from build123d import *

# Parameters (mm, degrees)
SKETCH_W             = 95
SKETCH_H             = 48
PAD_DEPTH            = 2
SKETCH001_W          = 95
SKETCH001_H          = 48
SKETCH001_W_2        = 91
SKETCH001_H_2        = 44
PAD001_DEPTH         = 18.5
SKETCH002_W          = 43.5
SKETCH002_H          = 20.5
POCKET_DEPTH         = 5
SKETCH003_W          = 5
SKETCH003_H          = 20.5
PAD002_DEPTH         = 2
SKETCH004_R          = 0.7
POCKET001_DEPTH      = 3
SKETCH005_W          = 4.5
SKETCH005_H          = 2.7
SKETCH005_W_2        = 5.5
SKETCH005_W_3        = 20
SKETCH005_H_2        = 2
SKETCH005_W_4        = 12
SKETCH005_H_3        = 1
SKETCH005_W_5        = 2
PAD003_DEPTH         = 2.5
PAD004_DEPTH         = 17
SKETCH007_W          = 1
SKETCH007_H          = 2.7
POCKET002_DEPTH      = 14
SKETCH008_W          = 3.5
SKETCH008_H          = 9.5
POCKET003_DEPTH      = 2
SKETCH009_R          = 1
POCKET004_DEPTH      = 2
PAD005_DEPTH         = 4
SKETCH011_W          = 70
SKETCH011_H          = 3
SKETCH011_W_2        = 2
SKETCH011_H_2        = 3.5
SKETCH011_W_3        = 3
PAD006_DEPTH         = 15
SKETCH012_W          = 15
SKETCH012_H          = 12.85
PAD007_DEPTH         = 7.3
SKETCH013_W          = 12
SKETCH013_H          = 10.8
POCKET005_DEPTH      = 4
SKETCH014_W          = 5
SKETCH014_H          = 5
POCKET006_DEPTH      = 6
SKETCH015_R          = 3.2
POCKET007_DEPTH      = 5
POCKET007_DEPTH_BACK = 100
SKETCH017_R          = 1
POCKET008_DEPTH      = 10
SKETCH018_R          = 1.6
POCKET009_DEPTH      = 5
SKETCH019_R          = 1.6
POCKET010_DEPTH      = 5
SKETCH026_R          = 2.1
SKETCH026_R_2        = 2.5
POCKET014_DEPTH      = 5
FILLET003_R          = 2
FILLET004_R          = 1.95
CHAMFER001_SIZE      = 2
FILLET005_R          = 1
CHAMFER003_SIZE      = 1.2
CHAMFER004_SIZE      = 1.2
FILLET013_R          = 1
FILLET014_R          = 0.9
SKETCH049_W          = 3
SKETCH049_H          = 1
POCKET020_DEPTH      = 2.5
SKETCH050_W          = 5
SKETCH050_H          = 7
POCKET021_DEPTH      = 5


with BuildPart() as part:
    # Sketch → Pad (new body)
    with BuildSketch(Plane.XY):
        with Locations((47.5, 24)):
            Rectangle(SKETCH_W, SKETCH_H)
    extrude(amount=PAD_DEPTH)

    # Sketch001 (on Face6 of Pad) → Pad001 (join)
    with BuildSketch(Plane.XY.offset(2)):
        with Locations((47.5, 24)):
            Rectangle(SKETCH001_W, SKETCH001_H)
        with Locations((47.5, 24)):
            Rectangle(SKETCH001_W_2, SKETCH001_H_2, mode=Mode.SUBTRACT)
    extrude(amount=PAD001_DEPTH)

    # Sketch002 (on Face15 of Pad001) → Pocket (cut)
    with BuildSketch(Plane.XY.offset(2)):
        with Locations((66.25, 35.75)):
            Rectangle(SKETCH002_W, SKETCH002_H)
    extrude(amount=-POCKET_DEPTH, mode=Mode.SUBTRACT)

    # Sketch003 (on Face15 of Pocket) → Pad002 (join)
    with BuildSketch(Plane.XY.offset(2)):
        with Locations((42, 35.75)):
            Rectangle(SKETCH003_W, SKETCH003_H)
        with Locations((90.5, 35.75)):
            Rectangle(SKETCH003_W, SKETCH003_H)
    extrude(amount=PAD002_DEPTH)

    # Sketch004 (on Face26 of Pad002) → Pocket001 (cut)
    with BuildSketch(Plane.XY.offset(4)):
        with Locations((90.2, 43.6)):
            Circle(SKETCH004_R)
        with Locations((90.2, 28.6)):
            Circle(SKETCH004_R)
        with Locations((42, 43.6)):
            Circle(SKETCH004_R)
        with Locations((42, 28.6)):
            Circle(SKETCH004_R)
    extrude(amount=-POCKET001_DEPTH, mode=Mode.SUBTRACT)

    # Sketch005 (on Face16 of Pocket001) → Pad003 (join)
    with BuildSketch(Plane.XY.offset(2)):
        with Locations((4.25, 44.65)):
            Rectangle(SKETCH005_W, SKETCH005_H)
        with Locations((19.25, 44.65)):
            Rectangle(SKETCH005_W_2, SKETCH005_H)
        with Locations((12, 40.6)):
            Rectangle(SKETCH005_W_3, SKETCH005_H_2)
        with Locations((8, 37.35)):
            Rectangle(SKETCH005_W_4, SKETCH005_H_3)
        with Locations((21, 37.35)):
            Rectangle(SKETCH005_W_5, SKETCH005_H_3)
    extrude(amount=PAD003_DEPTH)

    # Sketch006 (on Face16 of Pad003) → Pad004 (join)
    with BuildSketch(Plane.XY.offset(2)):
        Polygon((30, 46), (33, 46), (33, 36.85), (27.6, 36.85), (27.6, 40.6), (30, 40.6), align=None)
    extrude(amount=PAD004_DEPTH)

    # Sketch007 (on Face13 of Pad004) → Pocket002 (cut)
    with BuildSketch(Plane.XY.offset(20.5)):
        with Locations((1.5, 44.65)):
            Rectangle(SKETCH007_W, SKETCH007_H)
    extrude(amount=-POCKET002_DEPTH, mode=Mode.SUBTRACT)

    # Sketch008 (on Face7 of Pocket002) → Pocket003 (cut)
    with BuildSketch(Plane(origin=(0, 0, 0), x_dir=(0, -1, 0), z_dir=(-1, 0, 0))):
        with Locations((-44.25, 10.25)):
            Rectangle(SKETCH008_W, SKETCH008_H)
    extrude(amount=-POCKET003_DEPTH, mode=Mode.SUBTRACT)

    # Sketch009 (on Face14 of Pocket003) → Pocket004 (cut)
    with BuildSketch(Plane(origin=(0, 48, 0), x_dir=(-1, 0, 0), z_dir=(0, 1, 0))):
        with Locations((-9.2, 3)):
            Circle(SKETCH009_R)
        with Locations((-13.7, 3)):
            Circle(SKETCH009_R)
    extrude(amount=-POCKET004_DEPTH, mode=Mode.SUBTRACT)

    # Sketch010 (on Face20 of Pocket004) → Pad005 (join)
    with BuildSketch(Plane.XY.offset(2)):
        Polygon((2, 35.5), (20.5, 35.5), (20.5, 2), (22.5, 2), (22.5, 36.85), (20, 36.85), (20, 35.85), (14, 35.85), (14, 36.85), (2, 36.85), align=None)
    extrude(amount=PAD005_DEPTH)

    # Sketch011 (on Face20 of Pad005) → Pad006 (join)
    with BuildSketch(Plane.XY.offset(2)):
        with Locations((58, 22.5)):
            Rectangle(SKETCH011_W, SKETCH011_H)
        with Locations((92, 3.75)):
            Rectangle(SKETCH011_W_2, SKETCH011_H_2)
        with Locations((92, 19.25)):
            Rectangle(SKETCH011_W_2, SKETCH011_H_2)
        with Locations((24.5, 19.25)):
            Rectangle(SKETCH011_W_3, SKETCH011_H_2)
        with Locations((24.5, 3.75)):
            Rectangle(SKETCH011_W_3, SKETCH011_H_2)
    extrude(amount=PAD006_DEPTH)

    # Sketch012 (on Face20 of Pad006) → Pad007 (join)
    with BuildSketch(Plane.XY.offset(2)):
        with Locations((30, 30.425)):
            Rectangle(SKETCH012_W, SKETCH012_H)
    extrude(amount=PAD007_DEPTH)

    # Sketch013 (on Face73 of Pad007) → Pocket005 (cut)
    with BuildSketch(Plane.XY.offset(9.3)):
        with Locations((30.25, 30.425)):
            Rectangle(SKETCH013_W, SKETCH013_H)
    extrude(amount=-POCKET005_DEPTH, mode=Mode.SUBTRACT)

    # Sketch014 (on Face107 of Pocket005) → Pocket006 (cut)
    with BuildSketch(Plane.XY.offset(5.3)):
        with Locations((30.25, 30.425)):
            Rectangle(SKETCH014_W, SKETCH014_H)
    extrude(amount=-POCKET006_DEPTH, mode=Mode.SUBTRACT)

    # Sketch015 (on Face25 of Pocket006) → Pocket007 (cut, two sides)
    with BuildSketch(Plane.XY.offset(2)) as pocket007_sk:
        with Locations((36.1, 41.5)):
            Circle(SKETCH015_R)
    extrude(amount=-POCKET007_DEPTH, mode=Mode.SUBTRACT)
    extrude(pocket007_sk.sketch, amount=POCKET007_DEPTH_BACK, mode=Mode.SUBTRACT)

    # Sketch017 (on Face27 of Pocket007) → Pocket008 (cut)
    with BuildSketch(Plane.XY.offset(19)):
        with Locations((30.5, 38.7)):
            Circle(SKETCH017_R)
    extrude(amount=-POCKET008_DEPTH, mode=Mode.SUBTRACT)

    # Sketch018 (on Face5 of Pocket008) → Pocket009 (cut)
    with BuildSketch(Plane.XZ):
        with Locations((15, 17)):
            Circle(SKETCH018_R)
    extrude(amount=-POCKET009_DEPTH, mode=Mode.SUBTRACT)

    # Sketch019 (on Face8 of Pocket009) → Pocket010 (cut)
    with BuildSketch(Plane.YZ.offset(95)):
        with Locations((35, 17)):
            Circle(SKETCH019_R)
    extrude(amount=-POCKET010_DEPTH, mode=Mode.SUBTRACT)

    # Sketch026 (on Face7 of Pocket010) → Pocket014 (cut)
    with BuildSketch(Plane(origin=(0, 0, 0), x_dir=(0, -1, 0), z_dir=(-1, 0, 0))):
        with Locations((-11.5, 11.5)):
            Circle(SKETCH026_R)
        with Locations((-18.25, 11.5)):
            Circle(SKETCH026_R_2)
    extrude(amount=-POCKET014_DEPTH, mode=Mode.SUBTRACT)

    # Fillet003
    fillet003_edges = [part.edges().sort_by_distance(p)[0] for p in [
        (0, 0, 1),
        (95, 0, 11.25),
        (95, 48, 11.25),
    ]]
    fillet(fillet003_edges, radius=FILLET003_R)

    # Fillet004
    fillet004_edges = [part.edges().sort_by_distance(p)[0] for p in [
        (0, 48, 1),
    ]]
    fillet(fillet004_edges, radius=FILLET004_R)

    # Chamfer001
    chamfer001_edges = [part.edges().sort_by_distance(p)[0] for p in [
        (30.25, 27.925, 0),
        (32.75, 30.425, 0),
        (30.25, 32.925, 0),
        (27.75, 30.425, 0),
    ]]
    chamfer(chamfer001_edges, length=CHAMFER001_SIZE)

    # Fillet005
    fillet005_edges = [part.edges().sort_by_distance(p)[0] for p in [
        (47.475, 48, 0),
    ]]
    fillet(fillet005_edges, radius=FILLET005_R)

    # Chamfer003
    chamfer003_edges = [part.edges().sort_by_distance(p)[0] for p in [
        (95, 33.4, 17),
    ]]
    chamfer(chamfer003_edges, length=CHAMFER003_SIZE)

    # Chamfer004
    chamfer004_edges = [part.edges().sort_by_distance(p)[0] for p in [
        (13.4, 0, 17),
    ]]
    chamfer(chamfer004_edges, length=CHAMFER004_SIZE)

    # Fillet013
    fillet013_edges = [part.edges().sort_by_distance(p)[0] for p in [
        (6.5, 43.3, 3.25),
        (16.5, 43.3, 3.25),
        (22, 43.3, 3.25),
        (22, 39.6, 3.25),
    ]]
    fillet(fillet013_edges, radius=FILLET013_R)

    # Fillet014
    fillet014_edges = [part.edges().sort_by_distance(p)[0] for p in [
        (22, 41.6, 3.25),
        (37.5, 36.85, 5.65),
        (27.6, 40.6, 10.5),
        (26, 17.5, 9.5),
        (26, 5.5, 9.5),
        (91, 17.5, 9.5),
        (91, 5.5, 9.5),
        (23, 17.5, 9.5),
        (23, 5.5, 9.5),
        (22.5, 13, 6),
        (58.5, 21, 17),
        (26, 19.25, 17),
        (23, 19.25, 17),
        (23, 22.5, 17),
        (58, 24, 17),
        (23, 3.75, 17),
        (24.5, 5.5, 17),
        (26, 3.75, 17),
        (91, 19.25, 17),
        (91, 3.75, 17),
        (92, 5.5, 17),
    ]]
    fillet(fillet014_edges, radius=FILLET014_R)

    # Sketch049 (on Face36 of Fillet014) → Pocket020 (cut)
    with BuildSketch(Plane.XY.offset(4.5)):
        with Locations((3.5, 37.35)):
            Rectangle(SKETCH049_W, SKETCH049_H)
    extrude(amount=-POCKET020_DEPTH, mode=Mode.SUBTRACT)

    # Sketch050 (on Face30 of Pocket020) → Pocket021 (cut)
    with BuildSketch(Plane(origin=(30, 0, 0), x_dir=(0, -1, 0), z_dir=(-1, 0, 0))):
        with Locations((-43.5, 10.5)):
            Rectangle(SKETCH050_W, SKETCH050_H)
    extrude(amount=-POCKET021_DEPTH, mode=Mode.SUBTRACT)


solid = part.part
Here's how the part is built. I have some questions about the finished solid (model axes, mm). A direction names the side the tool comes from. Round coordinates to 2 decimals unless told otherwise and drop trailing zeros. Order: outer loops, then holes, each group sorted by start corner. A loop starts at its lowest first (then second) coordinate and runs counter-clockwise, first axis right, second up. Notation, with made-up numbers: (87, 61) -> (127, 61) arc R18 ccw to (127, 71) -> close; hole circle Ø6 at (-24, -38). An arc over 180 degrees is marked (long way). Use CSV: the item, a comma, the result in double quotes.
1. I need wall thicknesses on line 1 along Y through (x, z) = (59, 9.5); line 2 along Y through (x, z) = (30.5, 13.5); line 3 along Y through (x, z) = (36.1, 8.5) (3 decimals). Which ranges of each line are inside material? Lowest first, please.
Recorded:
line 1,"y = 0 to 2, 21 to 24, 46 to 48"
line 2,"y = 0 to 2, 21 to 24, 36.85 to 37.7, 39.7 to 41, 46 to 48"
line 3,"y = 0 to 2, 21 to 25.025, 35.825 to 36.85, 46 to 48"
2. Thinking about a two-plate mould opening in Z: for faces 1 (the face through (31, 41, 10)), 2 (the face through (19, 45, 4.5)), 3 (the face through (30, 35.825, 7)), 4 (the face through (31, 44, 7)), which applies, pulls with the +Z half, pulls with the -Z half, needs draft (parallel to the pull), parting line crosses it, or undercut?
Recorded:
face 1,"undercut"
face 2,"pulls with the +Z half"
face 3,"needs draft"
face 4,"undercut"
3. Which directions (+Z, -Z, +X, -X, +Y, -Y) give clear straight access to the entire face, cutting with the end or side of a thin tool? Please do faces 5 (the face through (0.57, 0.6, 10.89)), 6 (the face through (30.187, 26.939, 1.014)), 7 (the face through (44.5, 36, 2)), 8 (the face through (33, 39, 10)).
Recorded:
face 5,"+Z, -Z, -X, -Y"
face 6,"-Z"
face 7,"+Z, -Z"
face 8,"+Z"
4. I want a section at A-A on y = 11. List the corners of the cut face in (x, z) for me.
Recorded:
outline,"(0, 1) arc R1 ccw to (1, 0) -> (94, 0) arc R1 ccw to (95, 1) -> (95, 20.5) -> (93, 20.5) -> (93, 2) -> (22.5, 2) -> (22.5, 5.1) arc R0.9 ccw to (21.6, 6) -> (20.5, 6) -> (20.5, 2) -> (2, 2) -> (2, 9.46) -> (0, 9.46) -> close; (0, 13.54) -> (2, 13.54) -> (2, 20.5) -> (0, 20.5) -> close"
5. I'm going to push flat-ended pins straight in: P1, Ø1.6, axis at x = 30.5, y = 39.5, coming from the +Z side; P2, Ø4.5, axis at x = 52, y = 21.5, coming from the +Z side; P3, Ø1.6, axis at x = 12.5, y = 41, coming from the +Z side. Where does each tip first touch, or does it pass through?
Recorded:
P1,"stops at z = 19"
P2,"stops at z = 17"
P3,"stops at z = 4.5"
